from build123d import *

# Parameters (mm, degrees)
F1_DEPTH = 8
F2_R     = 2
F3_R     = 0.5
F4_R     = 5


with BuildPart() as f1:
    # F0 (on Top) → F1 (new body)
    with BuildSketch(Plane.XY):
        Polygon((0, 14), (0, 0), (-15, 2), (-15.396491, -0.973684), (5, -3.693216), (5, 19), (-5.383829, 19), (-15, 15.5), (-15, 14), align=None)
    extrude(amount=F1_DEPTH)

    # F2
    f2_edges = [f1.edges().sort_by_distance(p)[0] for p in [
        (0, 0, 4),
    ]]
    fillet(f2_edges, radius=F2_R)

    # F3
    f3_edges = [f1.edges().sort_by_distance(p)[0] for p in [
        (-15, 14, 4),
        (-15, 2, 4),
        (-15.396491, -0.973684, 4),
        (-15, 15.5, 4),
        (-5.383829, 19, 4),
        (0, 14, 4),
        (5, 19, 4),
    ]]
    fillet(f3_edges, radius=F3_R)

    # F4
    f4_edges = [f1.edges().sort_by_distance(p)[0] for p in [
        (5, -3.693216, 4),
    ]]
    fillet(f4_edges, radius=F4_R)


solid = f1.part
Could you check a few things on this model? Use its own coordinates, in mm. A direction names the side the tool comes from. Coordinates: 2 decimals unless noted, no trailing zeros. Write each loop counter-clockwise with the first axis right and the second up, starting at its lowest first coordinate (ties: lowest second). Pieces come first, ordered by that corner, then holes. Notation, with made-up numbers: (-29.75, 6) - (14.25, 6) arc R5 cw to (14.25, 11) - close; hole circle Ø11 at (72, 88). An arc over 180 degrees is marked (long way). Write item = value, one per line.
1) Suppose I cut it at C-C on x = -2. Please give me the cut outline in (y, z), plus the area to 3 significant figures.
Result set:
outline = (-2.76, 0) - (0.28, 0) - (0.28, 8) - (-2.76, 8) - close; (14, 0) - (19, 0) - (19, 8) - (14, 8) - close
area = 64.4 mm2
2) Suppose I cut it at A-A on y = 1. Please give me the cut outline in (x, z), plus the area to 3 significant figures.
Result set:
outline = (-15.13, 0) - (-7.5, 0) - (-7.5, 8) - (-15.13, 8) - close; (-0.47, 0) - (4.9, 0) - (4.9, 8) - (-0.47, 8) - close
area = 104 mm2
3) Suppose I cut it at D-D on y = 3.5. Please give me the cut outline in (x, z), plus the area to 3 significant figures.
Result set:
outline = (0, 0) - (5, 0) - (5, 8) - (0, 8) - close
area = 40.0 mm2
4) Please list where these lines run through material, in increasing order: line 1 (X direction, y = 5.25, z = 2.75); line 2 (Y direction, x = -6, z = 2.75); line 3 (Y direction, x = -5, z = 7.75). Write a range as [from, to].
Result set:
line_1 = [0, 5]
line_2 = [-2.23, 0.8], [14, 18.78]
line_3 = [-2.36, 0.67], [14, 19]
5) Suppose I cut it at B-B on z = 2. Please give me the cut outline in (x, y), plus the area to 3 significant figures.
Result set:
outline = (-15.33, -0.48) arc R0.5 ccw to (-14.9, -1.04) - (-0.66, -2.94) arc R5 ccw to (5, 2.02) - (5, 18.5) arc R0.5 ccw to (4.5, 19) - (-5.3, 19) arc R0.5 ccw to (-5.47, 18.97) - (-14.67, 15.62) arc R0.5 ccw to (-15, 15.15) - (-15, 14.5) arc R0.5 ccw to (-14.5, 14) - (-0.5, 14) arc R0.5 cw to (0, 13.5) - (0, 2.28) arc R2 cw to (-2.26, 0.3) - (-14.5, 1.93) arc R0.5 ccw to (-15.07, 1.5) - close
area = 210 mm2
6) Will these pins go through, and if not, where does the flat tip stop? pin 1 Ø4 at (x, z) = (-4.5, 3.5) entering from -Y; pin 2 Ø1 at (x, z) = (-7, 2.5) entering from -Y; pin 3 Ø0.7 at (y, z) = (14.5, 5.5) entering from -X.
Result set:
pin_1 = -2.69
pin_2 = -2.16
pin_3 = -15
7) We'd pull the mould along Y, two halves only. Please class faces 4 (the flat face through (1, 8, 8)), 5 (the flat face through (0, 8, 4)), 6 (the flat face through (-15.2, 0.5, 3.9)): +Y half, -Y half, draft (parallel to the pull), parting line (faces both ways), or undercut.
Result set:
face_4 = draft
face_5 = undercut
face_6 = +Y half
8) For faces 1 (the cylindrical face through (-0.66, 0.8, 4.06)), 2 (the flat face through (-8, 14, 4)), 3 (the flat face through (5, 10, 4)), which set-ups out of +Z, -Z, +X, -X, +Y, -Y let a thin tool reach every point of the face, with its end or its side?
Result set:
face_1 = +Z, -Z
face_2 = +Z, -Z, -X
face_3 = +Z, -Z, +X, +Y, -Y
